Could you check a few things on this model? Use its own coordinates, in mm. Face numbers are marked on the shaded views. Round coordinates to 2 decimals unless told otherwise and drop trailing zeros. Loops run counter-clockwise (first coordinate to the right, second up) from the corner with the lowest first, then second, coordinate; pieces in that order, holes last. Notation, with made-up numbers: (-18.5, 37) -> (14.5, 37) arc R10 cw to (14.5, 43) -> close; hole circle Ø1 at (45, 0.25). An arc over 180 degrees is marked (long way). One line per item, written item: value.
```python
from build123d import *

# Parameters (mm, degrees)
F0_R     = 3
F1_DEPTH = 10
F2_R     = 2
F3_DEPTH = 3
F4_R     = 3
F5_DEPTH = 8
F6_SIZE  = 0.4


with BuildPart() as f1:
    # F0 (on Front) → F1 (new body, symmetric)
    with BuildSketch(Plane.XZ):
        Circle(F0_R)
    extrude(amount=F1_DEPTH, both=True)

    # F2 (on face) → F3 (join)
    with BuildSketch(Plane.XZ.offset(10)):
        Circle(F2_R)
    extrude(amount=F3_DEPTH)

    # F4 (on face) → F5 (join)
    with BuildSketch(Plane.XZ.offset(13)):
        Circle(F4_R)
    extrude(amount=F5_DEPTH)

    # F6
    f6_edges = [f1.edges().sort_by_distance(p)[0] for p in [
        (-3, -21, 0),
    ]]
    chamfer(f6_edges, length=F6_SIZE)


solid = f1.part
```
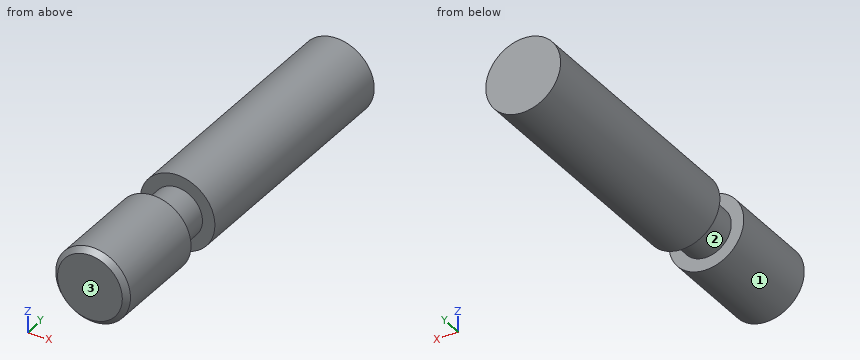
Item 1: I need wall thicknesses on line 1 (Y direction, x = 2.3, z = 0.55); line 2 (X direction, y = 5.5, z = 0.15); line 3 (Y direction, x = -2.65, z = -0.9). Which ranges of each line are inside material? Lowest first, please. Write a range as from..to.
Output:
line 1: y = -21..-13, -10..10
line 2: x = -3..3
line 3: y = -20.8..-13, -10..10
Item 2: If we section it at C-C on y = -9: List the corners of the cut face in (x, z) for me.
Output:
outline: circle Ø6 at (0, 0)
Item 3: If we section it at A-A on x = 0: List the corners of the cut face in (y, z) for me, plus the area to 3 significant figures.
Output:
outline: (-21, -2.6) -> (-20.6, -3) -> (-13, -3) -> (-13, -2) -> (-10, -2) -> (-10, -3) -> (10, -3) -> (10, 3) -> (-10, 3) -> (-10, 2) -> (-13, 2) -> (-13, 3) -> (-20.6, 3) -> (-21, 2.6) -> close
area: 180 mm²
Item 4: If we section it at B-B on z = 0: List the corners of the cut face in (x, y) for me, plus the area to 3 significant figures.
Output:
outline: (-3, -20.6) -> (-2.6, -21) -> (2.6, -21) -> (3, -20.6) -> (3, -13) -> (2, -13) -> (2, -10) -> (3, -10) -> (3, 10) -> (-3, 10) -> (-3, -10) -> (-2, -10) -> (-2, -13) -> (-3, -13) -> close
area: 180 mm²
Item 5: Will these pins go through, and if not, where does the flat tip stop? pin 1 Ø3 at (x, y) = (2.5, -7) entering from -Z; pin 2 Ø1 at (y, z) = (5, -1) entering from +X.
Output:
pin 1: stops at z = -2.83
pin 2: stops at x = 2.96
Item 6: If we mould it in two halves opening along Y, with no side actions, what happens to the marked faces 1, 2 and 3? For each: released by +Y, released by -Y, zero draft, split by the parting line, or undercut.
Output:
face 1: zero draft
face 2: undercut
face 3: released by -Y
